Read the model definition and answer for the solid it produces. Units are mm, in the model's axes. Give positions to 0.01 mm unless a question says otherwise; leave off trailing zeros. Write each loop counter-clockwise with the first axis right and the second up, starting at its lowest first coordinate (ties: lowest second). Pieces come first, ordered by that corner, then holes. Notation, with made-up numbers: (82.5, 8) -> (99.5, 8) arc R25 cw to (99.5, 23) -> close; hole circle Ø11 at (-36.75, 26). An arc over 180 degrees is marked (long way). Answer as CSV lines item,"result". Start each with the question number.
1. Find the intervals of material crossed by line 1 (Z direction, x = -1, y = -2.5); line 2 (Z direction, x = 4.75, y = -1); line 3 (X direction, y = -2.5, z = -2.25), in increasing order.
2. Given pin 1 (8 mm diameter, centred on x = 0.5, z = 4.5, fed in from -Y), flat-ended and moving along its own axis, determine where the tip first touches the part or whether it passes through.
3. For a pull along Z with two mould halves and no side action, classify faces 1 (the flat face through (4.8, -3, -8.2)), 2 (the flat face through (-9.5, -3, 0)), 3 (the cylindrical face through (4.918, -3.033, -2.039)), 4 (the flat face through (4.683, -3.042, 8.266)) as pulls with the +Z half, pulls with the -Z half, needs draft (parallel to the pull), parting line crosses it, or undercut.
4. The part is cut by section A-A, the plane z = 0. Determine the outline of the cut face in (x, y), and give its area (3 significant figures).
5. The part is cut by section B-B, the plane y = -3.5. Determine the outline of the cut face in (x, z).
Autodesk Inventor part; units mm, degrees
ref_plane "2CYL_XY" through (0, -3, 0) normal (0, 1, 0) x (1, 0, 0)
ref_plane "2CYL_YZ" through (0, -3, 0) normal (1, 0, 0) x (0, 0, -1)
ref_plane "2CYL_ZX" through (0, -3, 0) normal (0, 0, -1) x (0, 1, 0)
sketch "Sketch_1" plane through (0, 0, 0) normal (0, 0, 1) x (1, 0, 0)
  line L0 (0, -6) -> (0, 0)
  line L1 (0, 0) -> (9.45, 0)
  line L2 (9.45, 0) -> (20.6462, -3)
  line L3 (20.6462, -3) -> (9.45, -6)
  line L4 (9.45, -6) -> (0, -6)
  line L5 (0, -6) -> (0, 0)
revolve "Revolution1" add sketch "Sketch_1" angle 360 about axis through (0, -6, 0) along (0, 1, 0)
sketch "Sketch_2" plane through (0, 0, 0) normal (0, 1, 0) x (-1, 0, 0)
  line L0 (38, -38) -> (38, 38)
  line L1 (38, 38) -> (-38, 38)
  line L2 (-38, 38) -> (-38, -38)
  line L3 (-38, -38) -> (38, -38)
  line L4 (9.5, 5.4848) -> (0, 10.9697)
  line L5 (0, 10.9697) -> (-9.5, 5.4848)
  line L6 (-9.5, 5.4848) -> (-9.5, -5.4848)
  line L7 (-9.5, -5.4848) -> (0, -10.9697)
  line L8 (0, -10.9697) -> (9.5, -5.4848)
  line L9 (9.5, -5.4848) -> (9.5, 5.4848)
extrude "Extrusion1" cut sketch "Sketch_2" along normal mid plane 14
sketch "Sketch_3" plane through (0, 0, 0) normal (0, 0, 1) x (1, 0, 0)
  line L0 (0, -6) -> (0, 0)
  line L1 (0, 0) -> (6, 0)
  line L2 (6, 0) -> (5.3235, -0.6765)
  line L3 (5.3235, -0.6765) -> (5.3235, -5.3235)
  line L4 (5.3235, -5.3235) -> (6, -6)
  line L5 (6, -6) -> (0, -6)
  line L6 (0, -6) -> (0, 0)
revolve "Revolution2" cut sketch "Sketch_3" angle 360 about axis through (0, -6, 0) along (0, -1, 0)
thread "Thread1"
ref_plane "2CYL_XY" through (0, -3, 0) normal (0, 1, 0) x (1, 0, 0)
ref_plane "2CYL_YZ" through (0, -3, 0) normal (1, 0, 0) x (0, 0, -1)
ref_plane "2CYL_ZX" through (0, -3, 0) normal (0, 0, -1) x (0, 1, 0)
ref_plane "din439b_punkt_XY" through (0, 0, 0) normal (0, 1, 0) x (1, 0, 0)
ref_plane "din439b_punkt_YZ" through (0, 0, 0) normal (1, 0, 0) x (0, 0, -1)
ref_plane "din439b_punkt_ZX" through (0, 0, 0) normal (0, 0, -1) x (0, 1, 0)
properties part number "DIN-439-B - M12x1.25(F)"
Results found:
1,line 1,"z = -10.39 to -5.23, 5.23 to 10.39"
1,line 2,"z = -8.23 to -2.4, 2.4 to 8.23"
1,line 3,"x = -9.5 to -4.82, 4.82 to 9.5"
2,pin 1,"stops at y = -6"
3,face 1,"pulls with the -Z half"
3,face 2,"needs draft"
3,face 3,"undercut"
3,face 4,"pulls with the +Z half"
4,outline,"(-9.5, -5.99) -> (-9.45, -6) -> (-6, -6) -> (-5.32, -5.32) -> (-5.32, -0.68) -> (-6, 0) -> (-9.45, 0) -> (-9.5, -0.01) -> close; (5.32, -5.32) -> (6, -6) -> (9.45, -6) -> (9.5, -5.99) -> (9.5, -0.01) -> (9.45, 0) -> (6, 0) -> (5.32, -0.68) -> close"
4,area,"49.2 mm²"
5,outline,"(-9.5, -5.48) -> (0, -10.97) -> (9.5, -5.48) -> (9.5, 5.48) -> (0, 10.97) -> (-9.5, 5.48) -> close; hole circle Ø10.65 at (0, 0)"
